Here's the drawing with two shaded views (mm, measured from the low corner). I have some questions. A direction names the side the tool comes from. Round coordinates to 2 decimals unless told otherwise and drop trailing zeros. Loops run counter-clockwise (first coordinate to the right, second up) from the corner with the lowest first, then second, coordinate; pieces in that order, holes last.
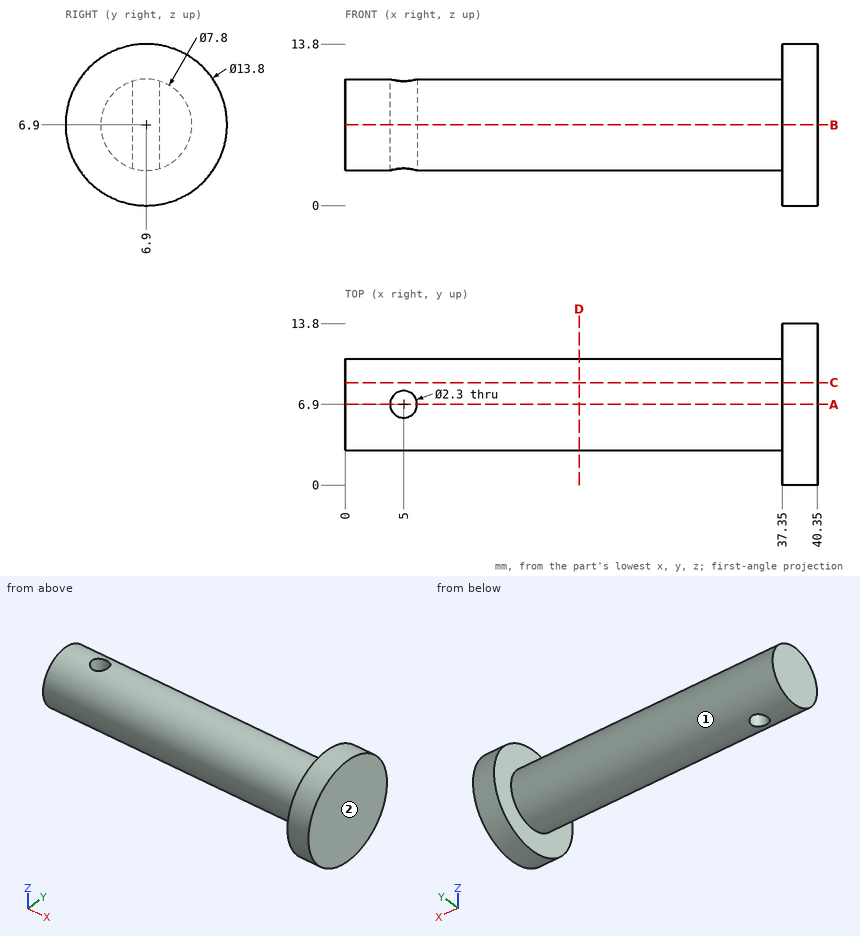
(1) Will these pins go through, and if not, where does the flat tip stop? P1, Ø1.5, axis at x = 18, z = 3.5, coming from the +Y side; P2, Ø6, axis at x = 6, y = 8, coming from the +Z side; P3, Ø2, axis at x = 7, z = 6, coming from the +Y side; P4, Ø1.5, axis at y = 11.5, z = 7, coming from the -X side.
Worked answers:
P1: stops at y = 9.76
P2: stops at z = 10.8
P3: stops at y = 10.8
P4: stops at x = 0
(2) For the marked faces 1 and 2, which set-ups out of +Z, -Z, +X, -X, +Y, -Y let a thin tool reach every point of the face, with its end or its side?
Worked answers:
face 1: -X
face 2: +Z, -Z, +X, +Y, -Y
(3) If we section it at D-D, the plane x = 20: List the corners of the cut face in (y, z) for me.
Worked answers:
outline: circle Ø7.8 at (6.9, 6.9)
(4) If we section it at B-B, the plane z = 6.9: List the corners of the cut face in (x, y) for me, then the cut area to 3 significant figures.
Worked answers:
outline: (0, 3) - (37.35, 3) - (37.35, 0) - (40.35, 0) - (40.35, 13.8) - (37.35, 13.8) - (37.35, 10.8) - (0, 10.8) - close; hole circle Ø2.3 at (5, 6.9)
area: 329 mm2
(5) If we section it at A-A, the plane y = 6.9: List the corners of the cut face in (x, z) for me, then the cut area to 3 significant figures.
Worked answers:
outline: (0, 3) - (3.85, 3) - (3.85, 10.8) - (0, 10.8) - close; (6.15, 3) - (37.35, 3) - (37.35, 0) - (40.35, 0) - (40.35, 13.8) - (37.35, 13.8) - (37.35, 10.8) - (6.15, 10.8) - close
area: 315 mm2
(6) If we section it at C-C, the plane y = 8.75: List the corners of the cut face in (x, z) for me.
Worked answers:
outline: (0, 3.47) - (37.35, 3.47) - (37.35, 0.25) - (40.35, 0.25) - (40.35, 13.55) - (37.35, 13.55) - (37.35, 10.33) - (0, 10.33) - close
(7) If I drill on line 1 (X direction, y = 6.9, z = 8.25); line 2 (X direction, y = 4, z = 1), over which ranges is the centre line in solid material (lowest first)?
Worked answers:
line 1: x = 0 to 3.85, 6.15 to 40.35
line 2: x = 37.35 to 40.35
